Part model, mm, in its own coordinate system. A direction names the side the tool comes from. Give positions to 0.01 mm unless a question says otherwise; leave off trailing zeros. Order: outer loops, then holes, each group sorted by start corner. A loop starts at its lowest first (then second) coordinate and runs counter-clockwise, first axis right, second up. Notation, with made-up numbers: M -24.75,-26 L -0.75,-26 A17 ccw -0.75,6 Z; hole C 30,-39.75 d7. An arc over 180 degrees is marked long. One line per question, with ' | ' between items.
Autodesk Inventor part; units mm, degrees
ref_plane "YZ Plane" through (0, 0, 0) normal (1, 0, 0) x (0, 1, 0)
ref_plane "XZ Plane" through (0, 0, 0) normal (0, 1, 0) x (-1, 0, 0)
ref_plane "XY Plane" through (0, 0, 0) normal (0, 0, 1) x (1, 0, 0)
sketch "CircuitBoard" plane through (0, 0, 0) normal (0, 0, 1) x (1, 0, 0)
  line L0 (-271.4625, 131.7625) -> (-267.0175, 131.7625) construction
  line L1 (0, 129.3813) -> (0, 5.9531)
  line L2 (0, 0) -> (-267.0175, 0) construction
  line L3 (-271.4625, 0) -> (-271.4625, 131.7625) construction
  line L4 (-271.4625, 95.25) -> (-267.0175, 95.25)
  line L5 (-267.0175, 95.25) -> (-267.0175, 86.1219) construction
  line L6 (-267.0175, 86.1219) -> (-271.4625, 86.1219)
  line L7 (-271.4625, 86.1219) -> (-271.4625, 95.25)
  line L8 (-271.4625, 95.25) -> (-262.3344, 95.25)
  line L9 (-262.3344, 95.25) -> (-262.3344, 86.1219)
  line L10 (-262.3344, 86.1219) -> (-271.4625, 86.1219)
  line L11 (-271.4625, 86.1219) -> (-271.4625, 95.25)
  line L12 (-267.0175, 95.25) -> (-267.0175, 129.3813)
  line L13 (-264.6363, 131.7625) -> (-2.3812, 131.7625)
  line L14 (-267.0175, 86.1219) -> (-267.0175, 5.9531)
  line L15 (-267.0175, 0) -> (-271.4625, 0) construction
  line L16 (-135.255, 0) -> (-140.0175, 0)
  line L17 (-140.0175, 0) -> (-140.0175, 3.5719)
  line L18 (-140.0175, 3.5719) -> (-135.255, 3.5719)
  line L19 (-135.255, 3.5719) -> (-135.255, 0)
  line L20 (-140.0175, 0) -> (-135.255, 0)
  line L21 (-135.255, 0) -> (-135.255, -1.5875)
  line L22 (-135.255, -1.5875) -> (-140.0175, -1.5875)
  line L23 (-140.0175, -1.5875) -> (-140.0175, 0)
  line L24 (-271.4625, 42.8625) -> (-267.0175, 42.8625)
  line L25 (-267.0175, 42.8625) -> (-267.0175, 38.1)
  line L26 (-267.0175, 38.1) -> (-271.4625, 38.1)
  line L27 (-271.4625, 38.1) -> (-271.4625, 42.8625)
  circle A0 centre (-262.8456, 127.5906) radius 1.7859
  arc A1 (-264.6363, 131.7625) -> (-267.0175, 129.3813) centre (-264.6362, 129.3813) ccw
  arc A2 (0, 129.3813) -> (-2.3812, 131.7625) centre (-2.3812, 129.3813) ccw
  circle A3 centre (-178.7081, 127.5906) radius 1.7859
  line L28 (-262.8456, 127.5906) -> (-178.7081, 127.5906) construction
  line L29 (-271.4625, 42.8625) -> (-273.05, 42.8625)
  line L30 (-273.05, 42.8625) -> (-273.05, 38.1)
  line L31 (-273.05, 38.1) -> (-271.4625, 38.1)
  line L32 (-271.4625, 38.1) -> (-271.4625, 42.8625)
  line L33 (-140.0175, 3.5719) -> (-264.6363, 3.5719)
  line L34 (-135.255, 3.5719) -> (-2.3813, 3.5719)
  line L35 (0, 3.5719) -> (0, 0) construction
  arc A4 (-267.0175, 5.9531) -> (-264.6363, 3.5719) centre (-264.6362, 5.9531) ccw
  arc A5 (-2.3813, 3.5719) -> (0, 5.9531) centre (-2.3813, 5.9531) ccw
  line L36 (-267.0175, 67.6672) -> (0, 67.6672) construction
  line L37 (-133.5087, 131.7625) -> (-133.5088, 3.5719) construction
  circle A6 centre (-4.1719, 127.5906) radius 1.7859
  circle A7 centre (-88.3094, 127.5906) radius 1.7859
  circle A8 centre (-262.8456, 7.7438) radius 1.7859
  circle A9 centre (-178.708, 7.7438) radius 1.7859
  circle A10 centre (-4.1719, 7.7438) radius 1.7859
  circle A11 centre (-88.3094, 7.7438) radius 1.7859
  point P0 (0, 131.7625)
  point P1 (-133.5088, 67.6672)
  dimension "d44" = 271.4625
  dimension "d45" = 131.7625
  dimension "d46" = 4.445
  dimension "d47" = 9.1281
  dimension "d48" = 36.5125
  dimension "d49" = 9.1281
  dimension "d50" = 131.7625
  dimension "d51" = 4.7625
  dimension "d52" = 3.5719
  dimension "d53" = 1.5875
  dimension "d54" = 4.7625
  dimension "d55" = 38.1
  dimension "d56" = 3.5719
  dimension "d57" = 4.1719
  dimension "d58" = 4.1719
  dimension "d59" = 2.3813
  dimension "d60" = 84.1375
  dimension "d61" = 1.5875
  dimension "d62" = 2.3813
  dimension "d65" = 88.3094
extrude "CircuitBoardFeature" add sketch "CircuitBoard" along normal blind 1.5875 contours L1 A5 L34 L18 L33 A4 L14 L10 L9 L8 L12 A1 L13 A2 | L19 L16 L17 L18 | L8 L9 L10 L6 L7 L4 | L26 L27 L24 L14
extrude "TopFeatures" add sketch "CircuitBoard" along normal blind 5.08 contours L19 L16 L17 L18 | L8 L9 L10 L6 L7 L4 | L26 L27 L24 L14
sketch "BottomProfile" plane through (0, 0, 0) normal (0, 0, -1) x (-1, 0, 0)
  line L0 (264.6363, 3.5719) -> (140.0175, 3.5719) construction
  line L1 (228.9175, 3.5719) -> (216.2175, 3.5719)
  line L2 (216.2175, 3.5719) -> (216.2175, 11.1919)
  line L3 (216.2175, 11.1919) -> (228.9175, 11.1919)
  line L4 (228.9175, 11.1919) -> (228.9175, 3.5719)
  line L5 (135.255, 3.5719) -> (2.3813, 3.5719) construction
  line L6 (50.8, 3.5719) -> (38.1, 3.5719)
  line L7 (38.1, 3.5719) -> (38.1, 11.1919)
  line L8 (38.1, 11.1919) -> (50.8, 11.1919)
  line L9 (50.8, 11.1919) -> (50.8, 3.5719)
  line L10 (0, 5.9531) -> (0, 129.3813) construction
  line L11 (0, 67.6672) -> (267.0175, 67.6672) construction
  line L12 (267.0175, 86.1219) -> (267.0175, 42.8625)
  line L13 (267.0175, 38.1) -> (267.0175, 5.9531)
  line L14 (228.9175, 131.7625) -> (216.2175, 131.7625)
  line L15 (216.2175, 131.7625) -> (216.2175, 124.1425)
  line L16 (216.2175, 124.1425) -> (228.9175, 124.1425)
  line L17 (228.9175, 124.1425) -> (228.9175, 131.7625)
  line L18 (50.8, 131.7625) -> (38.1, 131.7625)
  line L19 (38.1, 131.7625) -> (38.1, 124.1425)
  line L20 (38.1, 124.1425) -> (50.8, 124.1425)
  line L21 (50.8, 124.1425) -> (50.8, 131.7625)
  point P0 (0, 0)
  dimension "d70" = 38.1
  dimension "d71" = 38.1
  dimension "d72" = 12.7
  dimension "d73" = 7.62
extrude "BottomFeatures" add sketch "BottomProfile" along normal blind 1.5875
equation "\"d58\" = d57"
properties part number "seaboard-block-circuit-board"
1. Mould opens along X. For faces 1 (the flat face through (-267, 91, 5.08)), 2 (the flat face through (-271.462, 40, 3)) say: released by +X, released by -X, zero draft, split by the parting line, or undercut.
Worked out:
face 1: zero draft | face 2: released by -X
2. Tool access for faces 3 (the flat face through (-138, 0, 3)), 4 (the flat face through (-267, 86.122, 3)): list every direction of +Z, -Z, +X, -X, +Y, -Y with a clear straight run to the whole face (end or side of a thin tool).
Worked out:
face 3: +Z, -Z, +X, -X, -Y | face 4: +Z, -X
3. Slice it at A-A on z = 3.75. Give the number of separate pieces and of enclosed holes in the cut face, then the cut area to 3 significant figures.
Worked out:
separate pieces: 3 | enclosed holes: 0 | area: 122 mm2
4. Slice it at C-C on y = 114. Give the cut face in (x, z).
Worked out:
outline: M -267.02,0 L 0,0 L 0,1.59 L -267.02,1.59 Z
5. Slice it at D-D on x = -172. Give the cut face in (y, z).
Worked out:
outline: M 3.57,0 L 131.76,0 L 131.76,1.59 L 3.57,1.59 Z
6. Probe L1, parallel to Y at x = -49, z = 1.5; L2, parallel to Z at x = -166, y = 42.5; L3, parallel to X at y = 90, z = 2.75. List the from-to ranges inside material, lowest first. Write a range as from..to.
Worked out:
L1: y = 3.57..131.76 | L2: z = 0..1.59 | L3: x = -271.46..-262.33
7. Slice it at B-B on x = -222. Give the cut face in (y, z), then the cut area to 3 significant figures.
Worked out:
outline: M 3.57,-1.59 L 11.19,-1.59 L 11.19,0 L 124.14,0 L 124.14,-1.59 L 131.76,-1.59 L 131.76,1.59 L 3.57,1.59 Z | area: 228 mm2
8. Drop flat-ended pins along their axis: pin 1 (3 mm diameter, centred on y = 116, z = 0, fed in from -X); pin 2 (0.5 mm diameter, centred on y = 7.5, z = -0.5, fed in from +X); pin 3 (2 mm diameter, centred on x = -51.5, y = 95, fed in from -Z). Give the stop position or say it passes through.
Worked out:
pin 1: stops at x = -267.02 | pin 2: stops at x = -38.1 | pin 3: stops at z = 0
